Design review of the part built by this model. Coordinates are the model's own, in mm. A direction names the side the tool comes from. Coordinates: 2 decimals unless noted, no trailing zeros. Loops run counter-clockwise (first coordinate to the right, second up) from the corner with the lowest first, then second, coordinate; pieces in that order, holes last. Notation, with made-up numbers: M 16,75.5 L 60,75.5 A10 cw 60,82.5 Z; hole C 30,16 d1. An arc over 180 degrees is marked long. Put each result on its own line as item: value. Start each with the question number.
(1) Take a section at C-C, the plane x = -39.5. Give the boundary of the cut face in (y, z).
(2) Clearance check with flat-ended pins moving along their axes: pin 1 (1.2 mm diameter, centred on y = 49.5, z = 13, fed in from +X); pin 2 (1.5 mm diameter, centred on x = -14.5, z = -3, fed in from -Y); pin 3 (3.5 mm diameter, centred on x = -54, y = 41, fed in from -Z); pin 4 (0.8 mm diameter, centred on y = -39, z = -20, fed in from -X). State where each tip first meets the part, or that it passes through.
(3) For faces 1 (the flat face through (-54, 6, 20.5)), 2 (the flat face through (-54, 42, 18.5)), 3 (the flat face through (-55, -38.407, 21)), 4 (the flat face through (25.722, 0, -20)), 5 (the cylindrical face through (23.397, 40.128, -19.007)), list the 3-axis set-ups (+Z, -Z, +X, -X, +Y, -Y) from which the entire face can be reached by the end or side of a thin tool; tool diameter is ignored.
(4) Take a section at A-A, the plane y = -34. Give the boundary of the cut face in (x, z), then the cut area to 3 significant figures.
(5) The part is to be moulded in two halves that separate along Y. For faces 6 (the cylindrical face through (-55.663, 41.018, 19.007)), 7 (the flat face through (-15, 51.593, 0)), 8 (the flat face through (23, -39.407, -20)), say which applies: +Y half, -Y half, draft (parallel to the pull), parting line (faces both ways), or undercut.
(6) Take a section at B-B, the plane z = 8. Give the boundary of the cut face in (x, y).
(7) For probe 1 along Z at (x, y) = (-53, 19.5), list the stretches that pass through material, from the lowest coordinate up. Write a range as [from, to].
```python
from build123d import *

# Parameters (mm, degrees)
EXTRUDE_1_DEPTH = 1
SKETCH_2_R      = 1.5
EXTRUDE_2_DEPTH = 1
EXTRUDE_3_DEPTH = 1
SKETCH_4_R      = 1.5
EXTRUDE_5_DEPTH = 1
SKETCH_5_W      = 82
SKETCH_5_H      = 4
EXTRUDE_6_DEPTH = 0.5
SKETCH_6_W      = 21
SKETCH_6_H      = 4
EXTRUDE_7_DEPTH = 1
SKETCH_7_W      = 21
SKETCH_7_H      = 4
EXTRUDE_8_DEPTH = 1
SKETCH_8_W      = 6
SKETCH_8_H      = 4
EXTRUDE_9_DEPTH = 1


with BuildPart() as part:
    # Sketch 1 → Extrude 1 (new body)
    with BuildSketch(Plane(origin=(0, 0, -19.5), x_dir=(-1, 0, 0), z_dir=(0, 0, -1))):
        with BuildLine():
            Line((-21.722283328, 40.092812976), (-21.722283328, -38.407187024))
            Line((-21.722283328, -38.407187024), (-25.722283328, -38.407187024))
            Line((-25.722283328, -38.407187024), (-25.722283328, 40.092812976))
            ThreePointArc((-25.722283328, 40.092812976), (-26.222283328, 41.592812976), (-25.722283328, 43.092812976))
            Line((-25.722283328, 43.092812976), (-25.722283328, 51.592812976))
            Line((-25.722283328, 51.592812976), (-21.722283328, 51.592812976))
            Line((-21.722283328, 51.592812976), (-21.722283328, 43.092812976))
            ThreePointArc((-21.722283328, 43.092812976), (-21.222283328, 41.592812976), (-21.722283328, 40.092812976))
        make_face()
    extrude(amount=EXTRUDE_1_DEPTH)

    # Sketch 2 → Extrude 2 (add)
    with BuildSketch(Plane.XY.offset(-19.5)):
        with Locations((23.722283328, 41.592812976)):
            Circle(SKETCH_2_R)
    extrude(amount=EXTRUDE_2_DEPTH)



with BuildPart() as body_2:
    # Sketch 3 → Extrude 3 (new body)
    with BuildSketch(Plane.XY.offset(19.5)):
        with BuildLine():
            Line((-52.277716672, 40.092812976), (-52.277716672, -38.407187024))
            Line((-52.277716672, -38.407187024), (-56.277716672, -38.407187024))
            Line((-56.277716672, -38.407187024), (-56.277716672, 40.092812976))
            ThreePointArc((-56.277716672, 40.092812976), (-56.777716672, 41.592812976), (-56.277716672, 43.092812976))
            Line((-56.277716672, 43.092812976), (-56.277716672, 51.592812976))
            Line((-56.277716672, 51.592812976), (-52.277716672, 51.592812976))
            Line((-52.277716672, 51.592812976), (-52.277716672, 43.092812976))
            ThreePointArc((-52.277716672, 43.092812976), (-51.777716672, 41.592812976), (-52.277716672, 40.092812976))
        make_face()
    extrude(amount=EXTRUDE_3_DEPTH)

    # Sketch 4 → Extrude 5 (add)
    with BuildSketch(Plane(origin=(0, 0, 19.5), x_dir=(-1, 0, 0), z_dir=(0, 0, -1))):
        with Locations((54.277716672, 41.592812976)):
            Circle(SKETCH_4_R)
    extrude(amount=EXTRUDE_5_DEPTH)



with BuildPart() as body_3:
    # Sketch 5 → Extrude 6 (new body, symmetric)
    with BuildSketch(Plane.XY):
        with Locations((-15.277716672, 49.592812976)):
            Rectangle(SKETCH_5_W, SKETCH_5_H)
    extrude(amount=EXTRUDE_6_DEPTH, both=True)


with BuildPart() as body_2_1:
    add(body_2.part)

    add(body_3.part)  # Extrude 7 merges body 3
    # Sketch 6 → Extrude 7 (add)
    with BuildSketch(Plane.ZY.offset(56.277716672)):
        with Locations((10, 49.592812976)):
            Rectangle(SKETCH_6_W, SKETCH_6_H)
    extrude(amount=EXTRUDE_7_DEPTH)


with BuildPart() as part_1:
    add(part.part)

    add(body_2_1.part)  # Extrude 8 merges body 2
    # Sketch 7 → Extrude 8 (add)
    with BuildSketch(Plane(origin=(25.722283328, 0, 0), x_dir=(0, 0, -1), z_dir=(1, 0, 0))):
        with Locations((10, 49.592812976)):
            Rectangle(SKETCH_7_W, SKETCH_7_H)
    extrude(amount=EXTRUDE_8_DEPTH)

    # Sketch 8 → Extrude 9 (add)
    with BuildSketch(Plane.XZ.offset(38.407187024)):
        with Locations((-55.277716672, 20)):
            Rectangle(SKETCH_8_W, SKETCH_8_H)
        with Locations((22.722283328, -20)):
            Rectangle(SKETCH_8_W, SKETCH_8_H)
    extrude(amount=EXTRUDE_9_DEPTH)


solid = part_1.part
```
Computed values:
1. outline: M 47.59,-0.5 L 51.59,-0.5 L 51.59,0.5 L 47.59,0.5 Z
2. pin 1: stops at x = -56.28
2. pin 2: passes through
2. pin 3: stops at z = 18.5
2. pin 4: stops at x = 19.72
3. face 1: +Z, +X, -X, +Y
3. face 2: -Z, +X, -X, +Y
3. face 3: -X
3. face 4: +Z, -Z, +X, -Y
3. face 5: +Z
4. outline: M -56.28,19.5 L -52.28,19.5 L -52.28,20.5 L -56.28,20.5 Z; M 21.72,-20.5 L 25.72,-20.5 L 25.72,-19.5 L 21.72,-19.5 Z
4. area: 8.00 mm^2
5. face 6: undercut
5. face 7: +Y half
5. face 8: -Y half
6. outline: M -57.28,47.59 L -56.28,47.59 L -56.28,51.59 L -57.28,51.59 Z
7. probe 1: z = [19.5, 20.5]
